Could you check a few things on this model? Use its own coordinates, in mm. A direction names the side the tool comes from. Coordinates: 2 decimals unless noted, no trailing zeros. Order: outer loops, then holes, each group sorted by start corner. A loop starts at its lowest first (then second) coordinate and runs counter-clockwise, first axis right, second up.
```python
from build123d import *

# Parameters (mm, degrees)
SCHIZZO1_W                   = 34
SCHIZZO1_H                   = 39
ESTRUSIONE_ESTRUSIONE1_DEPTH = 10
SCHIZZO4_W                   = 32
SCHIZZO4_H                   = 37
ESTRUSIONE_ESTRUSIONE2_DEPTH = 2
SCHIZZO5_W                   = 30
SCHIZZO5_H                   = 35
TAGLIO_ESTRUSIONE2_DEPTH     = 11
RACCORDO1_R                  = 3
RACCORDO2_R                  = 0.75
TAGLIO_ESTRUSIONE3_REACH     = 47.879
SCHIZZO6_R                   = 5


with BuildPart() as part:
    # Schizzo1 → Estrusione-Estrusione1 (new body)
    with BuildSketch(Plane(origin=(0, 0, 0), x_dir=(1, 0, 0), z_dir=(0, 1, 0))):
        with Locations((-16.306007172, -9.682590788)):
            Rectangle(SCHIZZO1_W, SCHIZZO1_H)
    extrude(amount=ESTRUSIONE_ESTRUSIONE1_DEPTH)

    # Schizzo4 → Estrusione-Estrusione2 (add)
    with BuildSketch(Plane(origin=(0, 10, 0), x_dir=(1, 0, 0), z_dir=(0, 1, 0))):
        with Locations((-16.306007172, -9.682590788)):
            Rectangle(SCHIZZO4_W, SCHIZZO4_H)
    extrude(amount=ESTRUSIONE_ESTRUSIONE2_DEPTH)

    # Schizzo5 → Taglio-Estrusione2 (cut)
    with BuildSketch(Plane(origin=(0, 12, 0), x_dir=(1, 0, 0), z_dir=(0, 1, 0))):
        with Locations((-16.306007172, -9.682590788)):
            Rectangle(SCHIZZO5_W, SCHIZZO5_H)
    extrude(amount=-TAGLIO_ESTRUSIONE2_DEPTH, mode=Mode.SUBTRACT)

    # Raccordo1
    raccordo1_edges = [part.edges().sort_by_distance(p)[0] for p in [
        (-32.306007172, 11, -8.817409212),
        (-32.306007172, 11, 28.182590788),
        (-0.306007172, 11, 28.182590788),
        (-0.306007172, 11, -8.817409212),
        (-16.306007172, 0, -9.817409212),
        (0.693992828, 0, 9.682590788),
        (-16.306007172, 0, 29.182590788),
        (-33.306007172, 0, 9.682590788),
        (-33.306007172, 5, -9.817409212),
        (0.693992828, 5, -9.817409212),
        (0.693992828, 5, 29.182590788),
        (-33.306007172, 5, 29.182590788),
    ]]
    fillet(raccordo1_edges, radius=RACCORDO1_R)

    # Raccordo2
    raccordo2_edges = [part.edges().sort_by_distance(p)[0] for p in [
        (-31.306007172, 6.5, 27.182590788),
        (-31.306007172, 6.5, -7.817409212),
        (-1.306007172, 6.5, -7.817409212),
        (-1.306007172, 6.5, 27.182590788),
    ]]
    fillet(raccordo2_edges, radius=RACCORDO2_R)

    # Schizzo6 → Taglio-Estrusione3 (cut, up to next)
    with BuildSketch(Plane.XZ, mode=Mode.PRIVATE) as taglio_estrusione3_sk1:
        with Locations(Location((-16.306007172, 9.682590788, 0), (0, 0, 270))):
            Circle(SCHIZZO6_R)
    taglio_estrusione3_tool1 = extrude(taglio_estrusione3_sk1.sketch, amount=-TAGLIO_ESTRUSIONE3_REACH, mode=Mode.PRIVATE) & part.part
    add(taglio_estrusione3_tool1.solids().sort_by_distance((-16.306007, 0, 9.682591))[0], mode=Mode.SUBTRACT)


solid = part.part
```
Item 1: Suppose I cut it at C-C (y = 5). List the corners of the cut face in (x, z) for me, and give its area (3 significant figures).
Item 2: I need wall thicknesses on line 1 (X direction, y = 8.75, z = 14); line 2 (Z direction, x = -15, y = 3.5); line 3 (Z direction, x = -6, y = 10.75). Which ranges of each line are inside material? Lowest first, please.
Item 3: Thinking about a two-plate mould opening in X: for faces 1 (the face through (-21.187, 0.493, 10.766)), 2 (the face through (-0.21, 6.55, 28.33)), 3 (the face through (-33.306, 6, 10)), which applies, +X half, -X half, draft (parallel to the pull), parting line (faces both ways), or undercut?
Item 4: For pin 1 Ø1 at (y, z) = (11.5, 13.5) entering from +X; pin 2 Ø0.6 at (x, y) = (-11.5, 10.5) entering from +Z; pin 3 Ø1 at (x, y) = (-20.5, 11.5) entering from -Z, each with a flat end and sliding along its axis, tell me the tip position at first contact or that it passes through.
Item 5: Which directions (+Z, -Z, +X, -X, +Y, -Y) give clear straight access to the entire face, cutting with the end or side of a thin tool? Please do faces 4 (the face through (-31.306, 7, 10)), 5 (the face through (-0.306, 11, 10)), 6 (the face through (-1.21, 11.01, 27.33)).
Item 6: Suppose I cut it at A-A (z = 20.5). List the corners of the cut face in (x, y) for me, and give its area (3 significant figures).
Item 7: Suppose I cut it at D-D (z = 7). List the corners of the cut face in (x, y) for me.
Item 8: Suppose I cut it at B-B (x = -19.5). List the corners of the cut face in (y, z) for me.
Geometry results:
1. outline: (-33.31, -6.82) arc R3 ccw to (-30.31, -9.82) - (-2.31, -9.82) arc R3 ccw to (0.69, -6.82) - (0.69, 26.18) arc R3 ccw to (-2.31, 29.18) - (-30.31, 29.18) arc R3 ccw to (-33.31, 26.18) - close; hole (-31.31, -7.07) arc R0.75 ccw to (-30.56, -7.82) - (-2.06, -7.82) arc R0.75 ccw to (-1.31, -7.07) - (-1.31, 26.43) arc R0.75 ccw to (-2.06, 27.18) - (-30.56, 27.18) arc R0.75 ccw to (-31.31, 26.43) - close
1. area: 269 mm2
2. line 1: x = -33.31 to -31.31, -1.31 to 0.69
2. line 2: z = -9.82 to -7.82, 27.18 to 29.18
2. line 3: z = -8.82 to -7.82, 27.18 to 28.18
3. face 1: undercut
3. face 2: +X half
3. face 3: -X half
4. pin 1: stops at x = -0.31
4. pin 2: stops at z = 28.18
4. pin 3: stops at z = -8.82
5. face 4: +Y
5. face 5: +Z, -Z, +X, +Y
5. face 6: +Z, +X, +Y
6. outline: (-33.31, 3) arc R3 ccw to (-30.31, 0) - (-2.31, 0) arc R3 ccw to (0.69, 3) - (0.69, 10) - (-0.31, 10) - (-0.31, 12) - (-1.31, 12) - (-1.31, 1) - (-31.31, 1) - (-31.31, 12) - (-32.31, 12) - (-32.31, 10) - (-33.31, 10) - close
6. area: 70.1 mm2
7. outline: (-33.31, 3) arc R3 ccw to (-30.31, 0) - (-20.53, 0) - (-20.53, 1) - (-31.31, 1) - (-31.31, 12) - (-32.31, 12) - (-32.31, 10) - (-33.31, 10) - close; (-12.09, 0) - (-2.31, 0) arc R3 ccw to (0.69, 3) - (0.69, 10) - (-0.31, 10) - (-0.31, 12) - (-1.31, 12) - (-1.31, 1) - (-12.09, 1) - close
8. outline: (0, -6.82) arc R3 ccw to (3, -9.82) - (10, -9.82) - (10, -8.82) - (12, -8.82) - (12, -7.82) - (1, -7.82) - (1, 5.84) - (0, 5.84) - close; (0, 13.53) - (1, 13.53) - (1, 27.18) - (12, 27.18) - (12, 28.18) - (10, 28.18) - (10, 29.18) - (3, 29.18) arc R3 ccw to (0, 26.18) - close
